Source: CAD feature listing. Evaluate the final solid. Frame: model axes, mm. A direction names the side the tool comes from. Give positions to 0.01 mm unless a question says otherwise; leave off trailing zeros. Order: outer loops, then holes, each group sorted by start corner. A loop starts at its lowest first (then second) coordinate and runs counter-clockwise, first axis right, second up. Notation, with made-up numbers: M 86,-18 L 126,-18 A25 cw 126,18 Z; hole C -34,52 d11. An arc over 180 degrees is marked long. Return JSON: item names as keys, results as strings.
from build123d import *

# Parameters (mm, degrees)
F0_W     = 152.4
F0_H     = 76.2
F1_DEPTH = 76.2
F2_W     = 71.4375
F2_H     = 71.4375
F3_DEPTH = 152.4
F4_R     = 7.9375
F5_DEPTH = 4.7625
F6_R     = 7.9375
F7_DEPTH = 4.7625


with BuildPart() as f1:
    # F0 (on Right) → F1 (new body)
    with BuildSketch(Plane.YZ):
        with Locations((0, 7.474488)):
            Rectangle(F0_W, F0_H)
    extrude(amount=-F1_DEPTH)

    # F2 (on face) → F3 (cut)
    with BuildSketch(Plane(origin=(0, 76.2, 0), x_dir=(-1, 0, 0), z_dir=(0, 1, 0))):
        with Locations((40.48125, 5.093238)):
            Rectangle(F2_W, F2_H)
    extrude(amount=-F3_DEPTH, mode=Mode.SUBTRACT)

    # F4 (on face) → F5 (cut, through all)
    with BuildSketch(Plane.YZ):
        with Locations((-38.1, -5.225512)):
            Circle(F4_R)
        with Locations((38.1, -5.225512)):
            Circle(F4_R)
    extrude(amount=-F5_DEPTH, mode=Mode.SUBTRACT)

    # F6 (on face) → F7 (cut, through all)
    with BuildSketch(Plane.XY.offset(45.574488)):
        with Locations((-38.1, 50.8)):
            Circle(F6_R)
        with Locations((-38.1, -38.1)):
            Circle(F6_R)
    extrude(amount=-F7_DEPTH, mode=Mode.SUBTRACT)


solid = f1.part
1. Section query B-B (x = -36.5). Return loops of the section in (y, z).
Evaluation:
{"outline": "M -76.2,40.81 L -45.87,40.81 L -45.87,45.57 L -76.2,45.57 Z; M -30.33,40.81 L 43.03,40.81 L 43.03,45.57 L -30.33,45.57 Z; M 58.57,40.81 L 76.2,40.81 L 76.2,45.57 L 58.57,45.57 Z"}
2. Section query C-C (z = -11.5). Return loops of the section in (x, y), then the cut area to 3 significant figures.
Evaluation:
{"outline": "M -4.76,-76.2 L 0,-76.2 L 0,-42.96 L -4.76,-42.96 Z; M -4.76,-33.24 L 0,-33.24 L 0,33.24 L -4.76,33.24 Z; M -4.76,42.96 L 0,42.96 L 0,76.2 L -4.76,76.2 Z", "area": "633 mm^2"}
3. Section query D-D (y = -59). Return loops of the section in (x, z).
Evaluation:
{"outline": "M -76.2,40.81 L -4.76,40.81 L -4.76,-30.63 L 0,-30.63 L 0,45.57 L -76.2,45.57 Z"}
4. Draft query along Z for faces 3 (the face through (-2.35, -30.77, -8.27)), 4 (the face through (0, -1, 8)), 5 (the face through (-2.35, 30.17, -4.88)), 6 (the face through (-40, 1, 40.812)). Return one class per face: pulls with the +Z half, pulls with the -Z half, needs draft (parallel to the pull), parting line crosses it, or undercut.
Evaluation:
{"face 3": "undercut", "face 4": "needs draft", "face 5": "undercut", "face 6": "pulls with the -Z half"}
5. Set-up query: faces 1 (the face through (-4, 76.2, 24)), 2 (the face through (-4.763, 1, 5)). Return all of +Z, -Z, +X, -X, +Y, -Y with unobstructed straight access to the full face (end or side cutting, diameter ignored); none if empty.
Evaluation:
{"face 1": "+Z, -Z, +X, -X, +Y", "face 2": "-Z, -X, +Y, -Y"}
6. Ray query, probe 1 along Y at (x, z) = (-38, 43); probe 2 along Z at (x, y) = (-1.2, -38.1); probe 3 along Z at (x, y) = (-59, 69). Return the intervals inside material, ascending.
Evaluation:
{"probe 1": "y = -76.2 to -46.04, -30.16 to 42.86, 58.74 to 76.2", "probe 2": "z = -30.63 to -13.16, 2.71 to 45.57", "probe 3": "z = 40.81 to 45.57"}
7. Section query A-A (y = 38.1). Return loops of the section in (x, z).
Evaluation:
{"outline": "M -76.2,40.81 L -4.76,40.81 L -4.76,2.71 L 0,2.71 L 0,45.57 L -76.2,45.57 Z; M -4.76,-30.63 L 0,-30.63 L 0,-13.16 L -4.76,-13.16 Z"}
8. First-contact query: pin 1 (21.5 mm diameter, centred on x = -53.5, y = 22, fed in from -Z); pin 2 (12 mm diameter, centred on x = -13.5, z = -20, fed in from +Y); pin 3 (10 mm diameter, centred on y = -23, z = 0.5, fed in from -X). Flat tips, straight axial feed; report the tip coordinate or a pass-through.
Evaluation:
{"pin 1": "stops at z = 40.81", "pin 2": "passes through", "pin 3": "stops at x = -4.76"}
